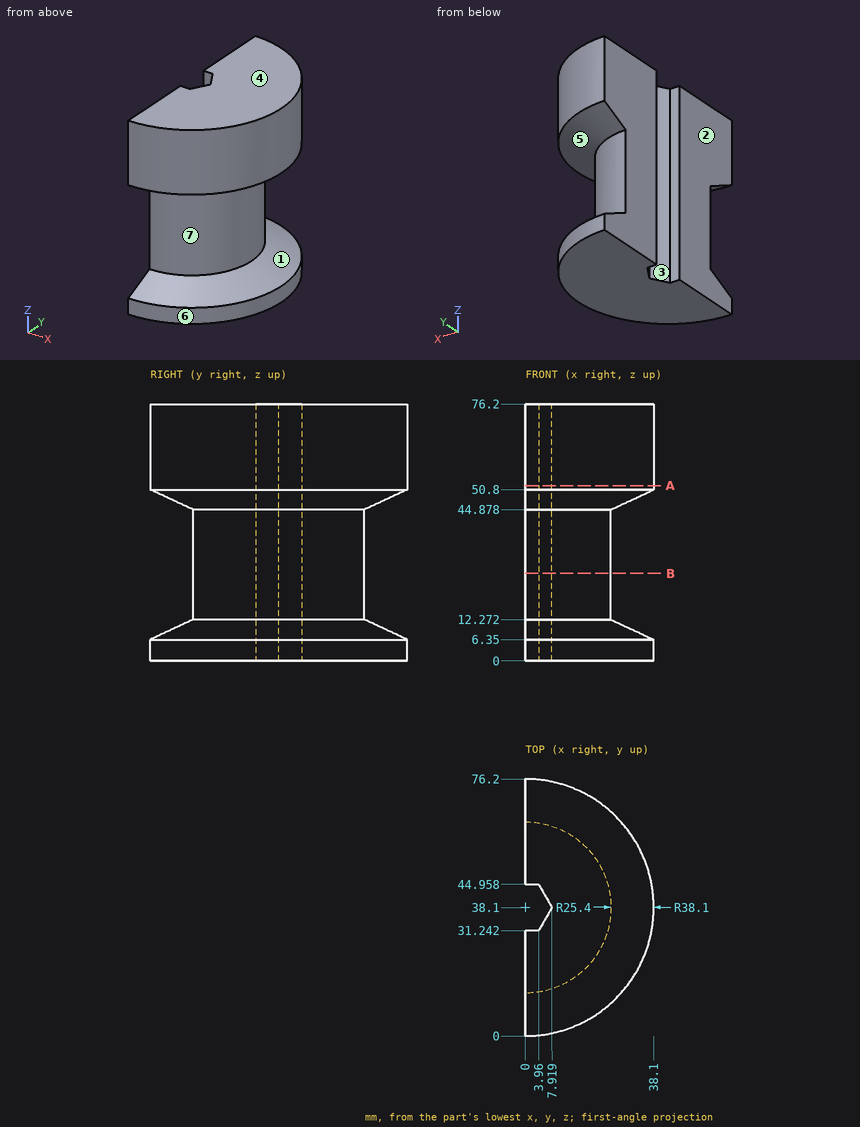
Can you work these out from the drawing? Everything is in mm from the part's minimum corner. A direction names the side the tool comes from. Coordinates: 2 decimals unless noted, no trailing zeros. Write each loop counter-clockwise with the first axis right and the second up, starting at its lowest first coordinate (ties: lowest second). Pieces come first, ordered by that corner, then holes. Notation, with made-up numbers: (39.25, -32) -> (70.25, -32) arc R19 ccw to (70.25, 5) -> close; hole circle Ø3 at (22, -9.75). An arc over 180 degrees is marked (long way). Write item = value, one per line.
(1) Imagine slicing it at B-B (z = 26). Please give me the cut outline in (x, y).
Verdict:
outline = (0, 12.7) arc R25.4 ccw to (0, 63.5) -> (0, 44.96) -> (3.96, 44.96) -> (7.92, 38.1) -> (3.96, 31.24) -> (0, 31.24) -> close
(2) For pin 1 (3 mm diameter, centred on x = 2, z = 46, fed in from -Y); pin 2 (1.2 mm diameter, centred on x = 2, z = 32, fed in from +Y); pin 3 (6 mm diameter, centred on x = 9, z = 32, fed in from +Y), each with a flat end and sliding along its axis, tell me the tip position at first contact or that it passes through.
Verdict:
pin_1 = 7.14
pin_2 = 63.46
pin_3 = 62.78
(3) If I drill on probe 1 along Z at (x, y) = (30.5, 23.5); probe 2 along Y at (x, z) = (2.5, 72.5); probe 3 along Z at (x, y) = (9.5, 7), over which ranges is the centre line in solid material (lowest first)?
Verdict:
probe_1 = 0 to 8.35, 48.8 to 76.2
probe_2 = 0.08 to 31.24, 44.96 to 76.12
probe_3 = 0 to 8.95, 48.2 to 76.2
(4) Thinking about a two-plate mould opening in Z: for the marked faces 4, 5, 6 and 7, which applies, +Z half, -Z half, draft (parallel to the pull), parting line (faces both ways), or undercut?
Verdict:
face_4 = +Z half
face_5 = undercut
face_6 = draft
face_7 = undercut
(5) On a 3-axis mill with a long thin cutter (end or side, diameter ignored), from which of +Z, -Z, +X, -X, +Y, -Y can I reach the whole of each face in a straight line? I mean the marked faces 1, 2 and 3. Say none if no direction works.
Verdict:
face_1 = +X
face_2 = +Z, -Z, -X, +Y, -Y
face_3 = +Z, -Z, -X
(6) Imagine slicing it at A-A (z = 52). Please give me the cut outline in (x, y), and give its area (3 significant figures).
Verdict:
outline = (0, 0) arc R38.1 ccw to (0, 76.2) -> (0, 44.96) -> (3.96, 44.96) -> (7.92, 38.1) -> (3.96, 31.24) -> (0, 31.24) -> close
area = 2,200 mm^2
